```python
from build123d import *

# Parameters (mm, degrees)
SKETCH_1_R          = 11
EXTRUDE_1_DEPTH     = 2.5
SKETCH_2_R          = 1
CUT_EXTRUDE_1_DEPTH = 3.5
FILLET_1_R          = 0.4
FILLET_2_R          = 1
SKETCH_3_R          = 9.5
SKETCH_3_R_2        = 1
EXTRUDE_2_DEPTH     = 0.5
FILLET_3_R          = 0.2


with BuildPart() as part:
    # 草图1 → 凸台-拉伸1 (new body)
    with BuildSketch(Plane(origin=(0, 0, 0), x_dir=(1, 0, 0), z_dir=(0, 1, 0))):
        Circle(SKETCH_1_R)
    extrude(amount=EXTRUDE_1_DEPTH)

    # 草图2 → 切除-拉伸1 (cut, through all)
    with BuildSketch(Plane(origin=(0, 2.5, 0), x_dir=(1, 0, 0), z_dir=(0, 1, 0))):
        Circle(SKETCH_2_R)
    extrude(amount=-CUT_EXTRUDE_1_DEPTH, mode=Mode.SUBTRACT)

    # 圆角1
    fillet_1_edges = [part.edges().sort_by_distance(p)[0] for p in [
        (-1, 2.5, 0),
    ]]
    fillet(fillet_1_edges, radius=FILLET_1_R)

    # 圆角2
    fillet_2_edges = [part.edges().sort_by_distance(p)[0] for p in [
        (-11, 2.5, 0),
    ]]
    fillet(fillet_2_edges, radius=FILLET_2_R)

    # 草图3 → 凸台-拉伸2 (add)
    with BuildSketch(Plane.XZ):
        Circle(SKETCH_3_R)
        Circle(SKETCH_3_R_2, mode=Mode.SUBTRACT)
    extrude(amount=EXTRUDE_2_DEPTH)

    # 圆角3
    fillet_3_edges = [part.edges().sort_by_distance(p)[0] for p in [
        (-9.5, 0, 0),
        (-9.5, -0.5, 0),
    ]]
    fillet(fillet_3_edges, radius=FILLET_3_R)


solid = part.part
```
Read the model definition and answer for the solid it produces. Units are mm, in the model's axes. A direction names the side the tool comes from. Give positions to 0.01 mm unless a question says otherwise; leave off trailing zeros. Write each loop counter-clockwise with the first axis right and the second up, starting at its lowest first coordinate (ties: lowest second). Pieces come first, ordered by that corner, then holes. Notation, with made-up numbers: (7, 1.5) - (17, 1.5) arc R12 cw to (17, 17.5) - close; hole circle Ø6 at (60.5, 45.25). An arc over 180 degrees is marked (long way). Write item = value, one per line. Start each with the question number.
Item 1: Find section A-A (x = 0). Give the vertices of the cut face in (y, z), then the cut area to 3 significant figures.
Item 2: Find section C-C (y = 0.35). Give the vertices of the cut face in (x, z), then the cut area to 3 significant figures.
Item 3: Find the intervals of material crossed by probe 1 along Z at (x, y) = (0, 1); probe 2 along Z at (x, y) = (-0.5, 0.4), in increasing order. Write a range as [from, to].
Item 4: Each of these flat-tipped pins is pushed along its axis until it touches: P1, Ø1.8, axis at x = 0, z = 0, coming from the -Y side; P2, Ø1.5, axis at x = 6.5, y = 2, coming from the +Z side. Where does it stop, or does it pass through?
Item 5: The mould has two halves that part along X. Classify faces 1 (the flat face through (2, -0.5, 0)), 2 (the cylindrical face through (0, 1, -1)), 3 (the cylindrical face through (-2.38, 0.74, 10.74)): +X half, -X half, draft (parallel to the pull), parting line (faces both ways), or undercut.
Item 6: A tool of negligible diameter and unlimited length cuts with its end or side. For faces 4 (the flat face through (0, 0, 10)), 5 (the flat face through (2, 2.5, 0)), from which of +Z, -Z, +X, -X, +Y, -Y can it reach the whole face along a straight path? Write none if from no direction.
Item 7: Find section B-B (z = 0). Give the vertices of the cut face in (x, y), then the cut area to 3 significant figures.
Response:
q1.outline = (-0.5, -9.3) arc R0.2 ccw to (-0.3, -9.5) - (-0.2, -9.5) arc R0.2 cw to (0, -9.7) - (0, -11) - (1.5, -11) arc R1 ccw to (2.5, -10) - (2.5, -1.4) arc R0.4 ccw to (2.1, -1) - (-0.5, -1) - close; (-0.5, 1) - (2.1, 1) arc R0.4 ccw to (2.5, 1.4) - (2.5, 10) arc R1 ccw to (1.5, 11) - (0, 11) - (0, 9.7) arc R0.2 cw to (-0.2, 9.5) - (-0.3, 9.5) arc R0.2 ccw to (-0.5, 9.3) - close
q1.area = 58.0 mm²
q2.outline = circle Ø22 at (0, 0); hole circle Ø2 at (0, 0)
q2.area = 377 mm²
q3.probe_1 = [-11, -1], [1, 11]
q3.probe_2 = [-10.99, -0.87], [0.87, 10.99]
q4.P1 = through
q4.P2 = 9.32
q5.face_1 = draft
q5.face_2 = undercut
q5.face_3 = parting line
q6.face_4 = -Y
q6.face_5 = +Z, -Z, +X, -X, +Y
q7.outline = (-11, 0) - (-9.7, 0) arc R0.2 cw to (-9.5, -0.2) - (-9.5, -0.3) arc R0.2 ccw to (-9.3, -0.5) - (-1, -0.5) - (-1, 2.1) arc R0.4 ccw to (-1.4, 2.5) - (-10, 2.5) arc R1 ccw to (-11, 1.5) - close; (1, -0.5) - (9.3, -0.5) arc R0.2 ccw to (9.5, -0.3) - (9.5, -0.2) arc R0.2 cw to (9.7, 0) - (11, 0) - (11, 1.5) arc R1 ccw to (10, 2.5) - (1.4, 2.5) arc R0.4 ccw to (1, 2.1) - close
q7.area = 58.0 mm²
